Design review of the part built by this model. Coordinates are the model's own, in mm. Coordinates: 2 decimals unless noted, no trailing zeros. Answer as a JSON object with one key per item and string values. Group by question number.
1. Consider section A-A (x = 9). Count the separate pieces of the cut face and the enclosed holes in it, then the cut area to 3 significant figures.
2. To check wall thickness, follow probe 1 along Z at (x, y) = (0, 1.35); probe 2 along Z at (x, y) = (0, 1.15); probe 3 along Z at (x, y) = (12, 1.5). State the ranges of each line that lie inside material, in increasing order.
3. Insertion check: pin 1 (12 mm diameter, centred on x = -13, z = -24, fed in from -Y); pin 2 (1 mm diameter, centred on y = 1, z = 17.5, fed in from -X); pin 3 (0.6 mm diameter, centred on x = 10.5, y = 1.5, fed in from +Z); pin 4 (1 mm diameter, centred on x = 1, y = 2, fed in from +Z). Each pin has a flat end and moves straight along its axis. Give the tip position at first contact, or say it passes through.
from build123d import *

# Parameters (mm, degrees)
F2_R     = 15
F2_R_2   = 3.5
F2_R_3   = 1.5
F3_DEPTH = 1000
F5_DEPTH = 2
F6_DEPTH = 10050


with BuildPart() as f1:
    # F0 (on Top) → F1 (revolve)
    with BuildSketch(Plane.XY):
        with BuildLine():
            Line((-30, 0), (0, 0))
            Line((0, 0), (0, 2))
            Line((0, 2), (-30, 2))
            add(Edge.make_bspline(
                [(-30, 2), (-30.4910149425, 1.5771952458), (-30.8094289155, 0.8702388721), (-30.4755121469, 0.4455515009), (-30, 0)],
                knots=[0, 0, 0, 0, 0.5130266248, 1, 1, 1, 1], degree=3))
        make_face()
    revolve(axis=Axis((0, 1, 0), (0, -1, 0)))

    # F2 (on Front) → F3 (cut)
    with BuildSketch(Plane.XZ):
        Circle(F2_R)
        Circle(F2_R_2, mode=Mode.SUBTRACT)
        Circle(F2_R_3)
    extrude(amount=-F3_DEPTH, mode=Mode.SUBTRACT)

    # F4 (on Front) → F5 (join)
    with BuildSketch(Plane.XZ):
        Polygon((-2.8139011922, 3.1256922416), (-9.7019712724, -12.3303449528), (-5.1349687969, -14.365655344), (-0.4918737939, -3.9470840711), (16.5167228414, -3.9470840711), (16.5167228414, 1.0529159289), (3.999228884, 1.0529159289), (-4.3775779681, 16.4923113486), (-8.7723915503, 14.1078588795), align=None)
    extrude(amount=-F5_DEPTH)

    # F2 (on Front) → F6 (cut)
    with BuildSketch(Plane.XZ):
        Circle(F2_R_3)
    extrude(amount=-F6_DEPTH, mode=Mode.SUBTRACT)


solid = f1.part
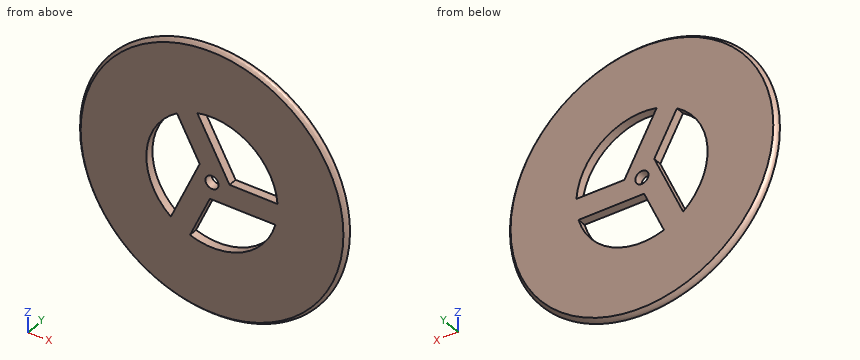
Findings below:
{
 "1": {"separate pieces": "3", "enclosed holes": "0", "area": "78.2 mm^2"},
 "2": {"probe 1": "z = -30.54 to -15, -3.95 to -1.5, 1.5 to 8.42, 15 to 30.54", "probe 2": "z = -30.62 to -15, -3.95 to -1.5, 1.5 to 8.42, 15 to 30.62", "probe 3": "z = -27.99 to -9, -3.95 to 1.05, 9 to 27.99"},
 "3": {"pin 1": "stops at y = 0", "pin 2": "stops at x = -25.5", "pin 3": "stops at z = 28.79", "pin 4": "stops at z = 30.44"}
}
